```python
from build123d import *

# Parameters (mm, degrees)
SALIENTE_EXTRUIR1_DEPTH = 3


with BuildPart() as part:
    # Model → Saliente-Extruir1 (new body)
    with BuildSketch(Plane.XY):
        with BuildLine():
            Line((66.714016933, 2.675368226), (68.538077011, 2.306726339))
            ThreePointArc((68.538077011, 2.306726339), (68.813397969, 2.426362589), (68.69376172, 2.701683548))
            Line((68.69376172, 2.701683548), (59.642778757, 9.23296694))
            Line((59.642778757, 9.23296694), (18.229236322, 26.798350869))
            Line((18.229236322, 26.798350869), (14.628932536, 28.325404932))
            ThreePointArc((14.628932536, 28.325404932), (16.425259576, 29.101436048), (18.375877707, 28.946181294))
            ThreePointArc((18.375877707, 28.946181294), (20.18694444, 29.13171328), (18.856885424, 30.37482544))
            ThreePointArc((18.856885424, 30.37482544), (15.51300149, 30.748167733), (12.514190479, 29.22236409))
            ThreePointArc((12.514190479, 29.22236409), (11.546461676, 30.101035899), (10.242109559, 30.186057881))
            ThreePointArc((10.242109559, 30.186057881), (9.413998041, 30.920271825), (8.310546545, 31.005322399))
            ThreePointArc((8.310546545, 31.005322399), (7.548095898, 31.654909282), (6.551125432, 31.751573638))
            ThreePointArc((6.551125432, 31.751573638), (5.898852104, 32.399314767), (4.980282277, 32.434790623))
            ThreePointArc((4.980282277, 32.434790623), (2.50269425, 34.859987429), (-0.691279819, 33.511450585))
            ThreePointArc((-0.691279819, 33.511450585), (-1.245238827, 31.123095112), (0.062521474, 29.0492399))
            ThreePointArc((0.062521474, 29.0492399), (0.732684306, 28.668767636), (1.483760549, 28.496251432))
            ThreePointArc((1.483760549, 28.496251432), (2.467023265, 28.521711274), (3.395589179, 28.846086231))
            ThreePointArc((3.395589179, 28.846086231), (4.04475241, 28.180155342), (4.973767828, 28.137644119))
            ThreePointArc((4.973767828, 28.137644119), (5.722549371, 27.472346961), (6.71729481, 27.354977378))
            ThreePointArc((6.71729481, 27.354977378), (7.529963713, 26.603706418), (8.63140861, 26.495734463))
            ThreePointArc((8.63140861, 26.495734463), (9.580661475, 25.59713434), (10.88296417, 25.485014428))
            ThreePointArc((10.88296417, 25.485014428), (11.803253278, 22.248656569), (14.350721609, 20.050623508))
            ThreePointArc((14.350721609, 20.050623508), (16.16662002, 19.920632003), (15.071202926, 21.374745554))
            ThreePointArc((15.071202926, 21.374745554), (13.631015332, 22.699462439), (12.978602224, 24.544285537))
            Line((12.978602224, 24.544285537), (16.546381847, 22.942714426))
            Line((16.546381847, 22.942714426), (57.585805628, 4.520176455))
            Line((57.585805628, 4.520176455), (66.714016933, 2.675368226))
        make_face()
    extrude(amount=SALIENTE_EXTRUIR1_DEPTH)


solid = part.part
```
Source: CAD feature listing. Evaluate the final solid. Frame: model axes, mm. Coordinates: 2 decimals unless noted, no trailing zeros. Order: outer loops, then holes, each group sorted by start corner. A loop starts at its lowest first (then second) coordinate and runs counter-clockwise, first axis right, second up. Notation, with made-up numbers: M 59.5,75.25 L 118.5,75.25 A26 ccw 118.5,114.25 Z; hole C 34,61.25 d5. An arc over 180 degrees is marked long. Write each question's results on one line, items separated by ' | '. Start each with the question number.
1) Section query B-B (x = 31). Return the cut outline in (y, z).
2) Draft query along X for faces 1 (the face through (-1.25, 31.16, 1.48)), 2 (the face through (4, 28.2, 1.5)), 3 (the face through (64.232, 5.922, 1.479)). Return one class per face: released by +X, released by -X, zero draft, split by the parting line, or undercut.
3) Section query C-C (y = 18). Return the cut outline in (x, z).
4) Section query A-A (z = 1.1). Return the cut outline in (x, y).
5) Line query: line 1 (Y direction, x = 15.5, z = 1.65); line 2 (Y direction, x = 20, z = 1.75); line 3 (Y direction, x = 17.5, z = 2.3). Output: solid intervals per line, ascending. Write a range as from..to.
6) Contact query for flat-ended pins moving along their axis: pin 1 Ø1 at (x, y) = (12.5, 26) entering from -Z; pin 2 Ø1.5 at (x, z) = (12, 1) entering from +Y. Output: stop coordinate, or through.
Answers:
1) outline: M 16.45,0 L 21.38,0 L 21.38,3 L 16.45,3 Z
2) face 1: released by -X | face 2: undercut | face 3: released by +X
3) outline: M 27.56,0 L 38.97,0 L 38.97,3 L 27.56,3 Z
4) outline: M -0.69,33.51 A3.18 ccw 0.06,29.05 A2.66 ccw 1.48,28.5 A3.18 ccw 3.4,28.85 A1.27 ccw 4.97,28.14 A1.67 ccw 6.72,27.35 A1.74 ccw 8.63,26.5 A1.98 ccw 10.88,25.49 A5.87 ccw 14.35,20.05 A1 ccw long 15.07,21.37 A4.06 cw 12.98,24.54 L 57.59,4.52 L 68.54,2.31 A0.21 ccw 68.69,2.7 L 59.64,9.23 L 14.63,28.33 A4.06 cw 18.38,28.95 A1 ccw long 18.86,30.37 A5.87 ccw 12.51,29.22 A1.98 ccw 10.24,30.19 A1.74 ccw 8.31,31.01 A1.67 ccw 6.55,31.75 A1.27 ccw 4.98,32.43 A3.13 ccw Z
5) line 1: y = 19.42..21.38, 23.41..27.96, 28.83..30.75 | line 2: y = 21.39..26.05, 28.8..30.1 | line 3: y = 22.51..27.11, 29.14..30.77
6) pin 1: stops at z = 0 | pin 2: stops at y = 30.2
